from build123d import *

# Parameters (mm, degrees)
F0_W      = 76.2
F0_H      = 38.1
F1_DEPTH  = 25.4
F2_R      = 6.35
F3_DEPTH  = 25.4
F4_R      = 6.35
F5_DEPTH  = 25.4
F6_R      = 6.35
F7_DEPTH  = 25.4
F8_R      = 6.35
F9_DEPTH  = 25.4
F10_R     = 13.692048
F11_DEPTH = 38.1
F12_W     = 12.7
F12_H     = 12.7


with BuildPart() as f1:
    # F0 (on Top) → F1 (new body)
    with BuildSketch(Plane.XY):
        with Locations((-8.536067, -11.700657)):
            Rectangle(F0_W, F0_H)
    extrude(amount=F1_DEPTH)

    # F2 (on Top) → F3 (cut)
    with BuildSketch(Plane.XY):
        with Locations((-39.016067, -0.270657)):
            Circle(F2_R)
    extrude(amount=F3_DEPTH, mode=Mode.SUBTRACT)

    # F4 (on Top) → F5 (cut)
    with BuildSketch(Plane.XY):
        with Locations((21.943933, -0.270657)):
            Circle(F4_R)
    extrude(amount=F5_DEPTH, mode=Mode.SUBTRACT)

    # F6 (on Top) → F7 (cut)
    with BuildSketch(Plane.XY):
        with Locations((-39.016067, -23.130657)):
            Circle(F6_R)
    extrude(amount=F7_DEPTH, mode=Mode.SUBTRACT)

    # F8 (on Top) → F9 (cut)
    with BuildSketch(Plane.XY):
        with Locations((21.943933, -23.130657)):
            Circle(F8_R)
    extrude(amount=F9_DEPTH, mode=Mode.SUBTRACT)

    # F10 (on face) → F11 (join)
    with BuildSketch(Plane.XY.offset(25.4)):
        with Locations((-9.878693, -10.635504)):
            Circle(F10_R)
    extrude(amount=F11_DEPTH)

    # F12 (on Front) → F13 (revolve, cut)
    with BuildSketch(Plane.XZ):
        with Locations((-25.066885, 39.424001)):
            Rectangle(F12_W, F12_H)
    revolve(axis=Axis((-9.878693, -10.635504, 63.5), (0, 0, 1)), mode=Mode.SUBTRACT)


solid = f1.part
Geometry check sheet. Reference: the model listing, model coordinates, mm. A direction names the side the tool comes from. Round coordinates to 2 decimals unless told otherwise and drop trailing zeros. Write each loop counter-clockwise with the first axis right and the second up, starting at its lowest first coordinate (ties: lowest second). Pieces come first, ordered by that corner, then holes. Notation, with made-up numbers: (58, 53) - (85, 53) arc R23 ccw to (85, 73) - close; hole circle Ø3 at (81.5, 2). An arc over 180 degrees is marked (long way). One line per item, written item: value.
1. Set-up check for faces 4 (the face through (-12.85, -24, 44.18)), 5 (the face through (-46.636, -12, 13)): record each of +Z, -Z, +X, -X, +Y, -Y from which the full face is reachable in a straight line by a thin tool's end or side.
The answers:
face 4: +Z
face 5: +Z, -Z, -X, +Y, -Y
2. Depth check by flat-ended pin: pin 1 Ø6 at (y, z) = (-5, 53) entering from -X; pin 2 Ø5 at (x, y) = (-32.5, -17.5) entering from -Z; pin 3 Ø5 at (x, y) = (13.5, -10) entering from +Z; pin 4 Ø3 at (y, z) = (-19, 40) entering from +X. Enter the tip coordinate at first touch or a pass-through.
The answers:
pin 1: stops at x = -23.31
pin 2: stops at z = 0
pin 3: stops at z = 25.4
pin 4: stops at x = 1.97
3. Cross-section at B-B on y = -21. Record the boundary of the cut face in (x, z), and give its area (3 significant figures).
The answers:
outline: (-46.64, 0) - (-45, 0) - (-45, 25.4) - (-46.64, 25.4) - close; (-33.03, 0) - (15.96, 0) - (15.96, 25.4) - (-0.93, 25.4) - (-0.93, 63.5) - (-18.83, 63.5) - (-18.83, 25.4) - (-33.03, 25.4) - close; (27.93, 0) - (29.56, 0) - (29.56, 25.4) - (27.93, 25.4) - close
area: 2,010 mm^2
4. Cross-section at C-C on z = 8. Record the boundary of the cut face in (x, y), and give its area (3 significant figures).
The answers:
outline: (-46.64, -30.75) - (29.56, -30.75) - (29.56, 7.35) - (-46.64, 7.35) - close; hole circle Ø12.7 at (-39.02, -23.13); hole circle Ø12.7 at (-39.02, -0.27); hole circle Ø12.7 at (21.94, -23.13); hole circle Ø12.7 at (21.94, -0.27)
area: 2,400 mm^2
5. Scan lines: L1, parallel to X at y = -3.5, z = 12; L2, parallel to Z at x = -3, y = -27; L3, parallel to X at y = -10.5, z = 59. Record each from-to range of solid material in increasing order.
The answers:
L1: x = -46.64 to -44.48, -33.55 to 16.48, 27.41 to 29.56
L2: z = 0 to 25.4
L3: x = -23.57 to 3.81
6. Cross-section at D-D on x = -14. Record the boundary of the cut face in (y, z).
The answers:
outline: (-30.75, 0) - (7.35, 0) - (7.35, 25.4) - (2.42, 25.4) - (2.42, 63.5) - (-23.69, 63.5) - (-23.69, 25.4) - (-30.75, 25.4) - close
7. Cross-section at A-A on x = 19. Record the boundary of the cut face in (y, z), and give its area (3 significant figures).
The answers:
outline: (-30.75, 0) - (-28.76, 0) - (-28.76, 25.4) - (-30.75, 25.4) - close; (-17.5, 0) - (-5.9, 0) - (-5.9, 25.4) - (-17.5, 25.4) - close; (5.36, 0) - (7.35, 0) - (7.35, 25.4) - (5.36, 25.4) - close
area: 396 mm^2
8. Mould release check, pull along X, two halves, no side actions. Record for faces 1 (the face through (-44.06, -26.99, 12.52)), 2 (the face through (29.564, -12, 13)), 3 (the face through (-9, -30.751, 13)): released by +X, released by -X, zero draft, split by the parting line, or undercut.
The answers:
face 1: undercut
face 2: released by +X
face 3: zero draft
